Here's the drawing with two shaded views (mm, measured from the low corner). I have some questions. Coordinates: 2 decimals unless noted, no trailing zeros. Loops run counter-clockwise (first coordinate to the right, second up) from the corner with the lowest first, then second, coordinate; pieces in that order, holes last.
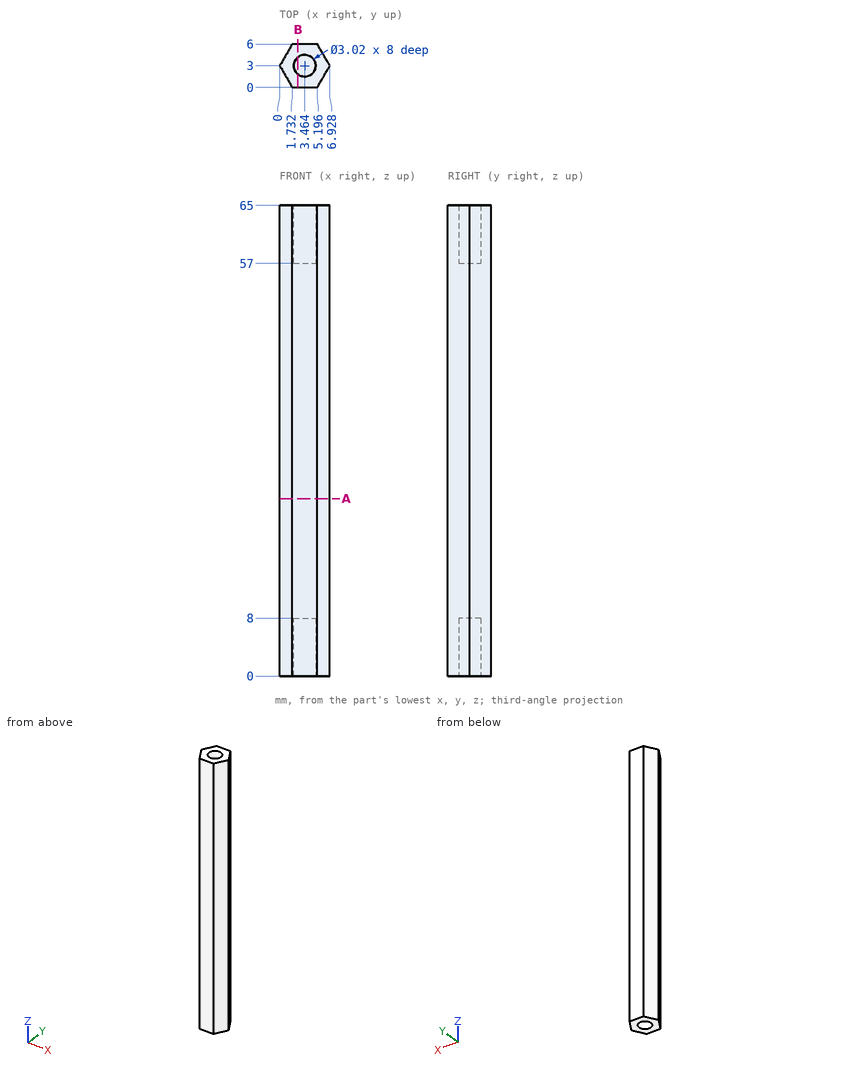
(1) I want a section at B-B on x = 2.5. Write out the boundary of the cut face in (y, z).
Check values:
outline: (0, 0) - (1.84, 0) - (1.84, 8) - (4.16, 8) - (4.16, 0) - (6, 0) - (6, 65) - (4.16, 65) - (4.16, 57) - (1.84, 57) - (1.84, 65) - (0, 65) - close
(2) I'm going to push a flat-ended pin straight in: pin 1 (2 mm diameter, centred on y = 3.5, z = 27, fed in from -X). Where does the tip first touch, or does it pass through?
Check values:
pin 1: stops at x = 0
(3) I want a section at A-A on z = 24.5. Write out the boundary of the cut face in (x, y), then the cut area to 3 significant figures.
Check values:
outline: (0, 3) - (1.73, 0) - (5.2, 0) - (6.93, 3) - (5.2, 6) - (1.73, 6) - close
area: 31.2 mm2
(4) If I drill on probe 1 along Y at (x, z) = (3.5, 5.5); probe 2 along Z at (x, y) = (3.5, 2.5); probe 3 along Y at (x, z) = (0.5, 15.5) (1 decimal), over which ranges is the centre line in solid material (lowest first)?
Check values:
probe 1: y = 0 to 1.49, 4.51 to 6
probe 2: z = 8 to 57
probe 3: y = 2.1 to 3.9
